Autodesk Inventor part; units mm, degrees
ref_plane "YZ Plane" through (0, 0, 0) normal (1, 0, 0) x (0, 1, 0)
ref_plane "XZ Plane" through (0, 0, 0) normal (0, 1, 0) x (-1, 0, 0)
ref_plane "XY Plane" through (0, 0, 0) normal (0, 0, 1) x (1, 0, 0)
sketch "Sketch1" plane through (0, 0, 0) normal (0, 1, 0) x (-1, 0, 0)
  line L0 (0, 0) -> (136.7536, 0)
  line L1 (136.7536, 0) -> (136.7536, -77.5208)
  line L2 (136.7536, -77.5208) -> (96.5708, -77.5208)
  line L3 (77.5208, -96.5708) -> (77.5208, -136.7536)
  line L4 (77.5208, -136.7536) -> (0, -136.7536)
  line L5 (0, -136.7536) -> (0, 0)
  arc A0 (96.5708, -77.5208) -> (77.5208, -96.5708) centre (96.5708, -96.5708) ccw
  circle A1 centre (9.525, -24.765) radius 2.2225
  circle A2 centre (24.765, -9.525) radius 2.2225
  circle A3 centre (9.525, -113.8936) radius 2.2225
  circle A4 centre (113.8936, -9.525) radius 2.2225
  circle A5 centre (126.5936, -44.45) radius 2.2225
  circle A6 centre (98.6536, -57.15) radius 2.2225
  circle A7 centre (92.3036, -21.59) radius 2.2225
  circle A8 centre (44.45, -126.5936) radius 2.2225
  circle A9 centre (57.15, -98.6536) radius 2.2225
  circle A10 centre (21.59, -92.3036) radius 2.2225
  line L6 (0, 0) -> (96.5708, -96.5708) construction
  dimension "d0" = 136.7536
  dimension "d1" = 77.5208
  dimension "d2" = 19.05
  dimension "d3" = 9.525
  dimension "d6" = 9.525
  dimension "d7" = 22.86
  dimension "d8" = 10.16
  dimension "d9" = 44.45
  dimension "d10" = 4.445
  dimension "d11" = 24.765
  dimension "d12" = 38.1
  dimension "d13" = 57.15
  dimension "d14" = 21.59
  dimension "d15" = 44.45
extrude "Extrusion1" add sketch "Sketch1" along normal blind 0.889
ref_plane "Work Plane1" through (0, 0, 0) normal (0.7071, 0, -0.7071) x (-0.7071, 0, -0.7071)
properties part number "NickBracket"
Input: part model. Units: mm. Frame: model coordinates. Give positions to 0.01 mm unless a question says otherwise; leave off trailing zeros. Loops run counter-clockwise (first coordinate to the right, second up) from the corner with the lowest first, then second, coordinate; pieces in that order, holes last. Notation, with made-up numbers: (60.5, 80) -> (79.5, 80) arc R12 cw to (79.5, 84) -> close; hole circle Ø5 at (-34.75, 69). An arc over 180 degrees is marked (long way). Use a Markdown table: item, result.
Q1. Section query D-D, the plane y = 0.65. State how many separate pieces and enclosed holes the cut face has, plus the area to 3 significant figures.
Entries:
| item | result |
|---|---|
| separate pieces | 1 |
| enclosed holes | 10 |
| area | 15,100 mm² |
Q2. Section query C-C, the plane x = -9.5. Return the cut outline in (y, z), plus the area to 3 significant figures.
Entries:
| item | result |
|---|---|
| outline | (0, -136.75) -> (0.89, -136.75) -> (0.89, -116.12) -> (0, -116.12) -> close; (0, -111.67) -> (0.89, -111.67) -> (0.89, -26.99) -> (0, -26.99) -> close; (0, -22.54) -> (0.89, -22.54) -> (0.89, 0) -> (0, 0) -> close |
| area | 114 mm² |
Q3. Ray query, probe 1 along Z at (x, y) = (-21.59, 0.3); probe 2 along Z at (x, y) = (-117, 0.65); probe 3 along X at (y, z) = (0.75, -9). Return the intervals inside material, ascending. Write a range as from..to.
Entries:
| item | result |
|---|---|
| probe 1 | z = -136.75..-94.53, -90.08..0 |
| probe 2 | z = -77.52..0 |
| probe 3 | x = -136.75..-116.05, -111.73..-26.92, -22.61..0 |
Q4. Section query B-B, the plane z = -44.45. Return the cut outline in (x, y), plus the area to 3 significant figures.
Entries:
| item | result |
|---|---|
| outline | (-136.75, 0) -> (-128.82, 0) -> (-128.82, 0.89) -> (-136.75, 0.89) -> close; (-124.37, 0) -> (0, 0) -> (0, 0.89) -> (-124.37, 0.89) -> close |
| area | 118 mm² |
Q5. Section query A-A, the plane x = -44.45. Return the cut outline in (y, z), plus the area to 3 significant figures.
Entries:
| item | result |
|---|---|
| outline | (0, -136.75) -> (0.89, -136.75) -> (0.89, -128.82) -> (0, -128.82) -> close; (0, -124.37) -> (0.89, -124.37) -> (0.89, 0) -> (0, 0) -> close |
| area | 118 mm² |
Q6. Pull-direction query (X, two-part tool) for faces 1 (the cylindrical face through (-83, 0.4, -83.2)), 2 (the flat face through (-52, 0, -52)), 3 (the cylindrical face through (-9.043, 0.438, -111.724)); classes: pulls with the +X half, pulls with the -X half, needs draft (parallel to the pull), parting line crosses it, or undercut.
Entries:
| item | result |
|---|---|
| face 1 | pulls with the -X half |
| face 2 | needs draft |
| face 3 | undercut |
